```python
from build123d import *

# Parameters (mm, degrees)
SKETCH1_R           = 5
BOSS_EXTRUDE1_DEPTH = 3.499993
SKETCH2_R           = 5.715
BOSS_EXTRUDE2_DEPTH = 0.500507
CUT_EXTRUDE1_REACH  = 11.018
SKETCH3_R           = 1.5


with BuildPart() as part:
    # Sketch1 → Boss-Extrude1 (new body)
    with BuildSketch(Plane(origin=(0, 0, 0), x_dir=(1, 0, 0), z_dir=(0, 1, 0))):
        with Locations(Location((0, 0, 0), (0, 0, 270))):
            Circle(SKETCH1_R)
    extrude(amount=BOSS_EXTRUDE1_DEPTH)

    # Sketch2 → Boss-Extrude2 (add)
    with BuildSketch(Plane(origin=(0, 3.499993, 0), x_dir=(1, 0, 0), z_dir=(0, 1, 0))):
        with Locations(Location((0, 0, 0), (0, 0, 270))):
            Circle(SKETCH2_R)
    extrude(amount=BOSS_EXTRUDE2_DEPTH)

    # Sketch3 → Cut-Extrude1 (cut, up to next)
    with BuildSketch(Plane(origin=(0, 4.0005, 0), x_dir=(1, 0, 0), z_dir=(0, 1, 0)), mode=Mode.PRIVATE) as cut_extrude1_sk1:
        with Locations(Location((0, 0, 0), (0, 0, 270))):
            Circle(SKETCH3_R)
    cut_extrude1_tool1 = extrude(cut_extrude1_sk1.sketch, amount=-CUT_EXTRUDE1_REACH, mode=Mode.PRIVATE) & part.part
    add(cut_extrude1_tool1.solids().sort_by_distance((0, 4.0005, 0))[0], mode=Mode.SUBTRACT)


solid = part.part
```
Geometry: final body of the model. Coordinates: model frame, mm. A direction names the side the tool comes from. Give positions to 0.01 mm unless a question says otherwise; leave off trailing zeros. Loops run counter-clockwise (first coordinate to the right, second up) from the corner with the lowest first, then second, coordinate; pieces in that order, holes last. Notation, with made-up numbers: (-27, -24.75) -> (28, -24.75) arc R15 ccw to (28, -5.75) -> close; hole circle Ø1 at (59.25, 57.25). An arc over 180 degrees is marked (long way). Use CSV: the item, a comma, the result in double quotes.
(1) Cut plane B-B (z = 0). Output: boundary loops of the cut face in (x, y) (1 decimal), plus the area to 3 significant figures.
From the geometry:
outline,"(-5.7, 3.5) -> (-5, 3.5) -> (-5, 0) -> (-1.5, 0) -> (-1.5, 4) -> (-5.7, 4) -> close; (1.5, 0) -> (5, 0) -> (5, 3.5) -> (5.7, 3.5) -> (5.7, 4) -> (1.5, 4) -> close"
area,"28.7 mm^2"
(2) Pull-direction query (Z, two-part tool) for faces 3 (the face through (-4.88, 1.73, -1.08)), 4 (the face through (0.45, 2.03, 1.43)), 5 (the face through (-1.2, 4, 1.2)); classes: released by +Z, released by -Z, zero draft, split by the parting line, or undercut.
From the geometry:
face 3,"split by the parting line"
face 4,"undercut"
face 5,"zero draft"
(3) Cut plane C-C (z = -3.5). Output: boundary loops of the cut face in (x, y), plus the area to 3 significant figures.
From the geometry:
outline,"(-4.52, 3.5) -> (-3.57, 3.5) -> (-3.57, 0) -> (3.57, 0) -> (3.57, 3.5) -> (4.52, 3.5) -> (4.52, 4) -> (-4.52, 4) -> close"
area,"29.5 mm^2"
(4) Cut plane A-A (x = 0). Output: boundary loops of the cut face in (y, z) (1 decimal).
From the geometry:
outline,"(0, -5) -> (3.5, -5) -> (3.5, -5.7) -> (4, -5.7) -> (4, -1.5) -> (0, -1.5) -> close; (0, 1.5) -> (4, 1.5) -> (4, 5.7) -> (3.5, 5.7) -> (3.5, 5) -> (0, 5) -> close"
(5) Access query for faces 1 (the face through (-5, 3.5, 2)), 2 (the face through (5.666, 3.747, -0.744)). Directions: +Z, -Z, +X, -X, +Y, -Y. A direction counts if a zero-diameter tool reaches every point of the face in a straight line with its end or side. Return the directions, or none.
From the geometry:
face 1,"-Y"
face 2,"+Y, -Y"
(6) Cut plane D-D (y = 1.65). Output: boundary loops of the cut face in (x, z).
From the geometry:
outline,"circle Ø10 at (0, 0); hole circle Ø3 at (0, 0)"
(7) Ray query, line 1 along X through (y, z) = (0.4, 0); line 2 along Y through (x, z) = (1.25, 5.25); line 3 along Z through (x, y) = (-1, 0.6). Return the intervals inside material, ascending. Write a range as [from, to].
From the geometry:
line 1,"[-5, -1.5], [1.5, 5]"
line 2,"[3.5, 4]"
line 3,"[-4.9, -1.12], [1.12, 4.9]"
(8) First-contact query: P1, Ø1.5, axis at x = 2, y = 0.5, coming from the -Z side. Flat tip, straight axial feed; report the tip coordinate or a pass-through.
From the geometry:
P1,"z = -4.84"
